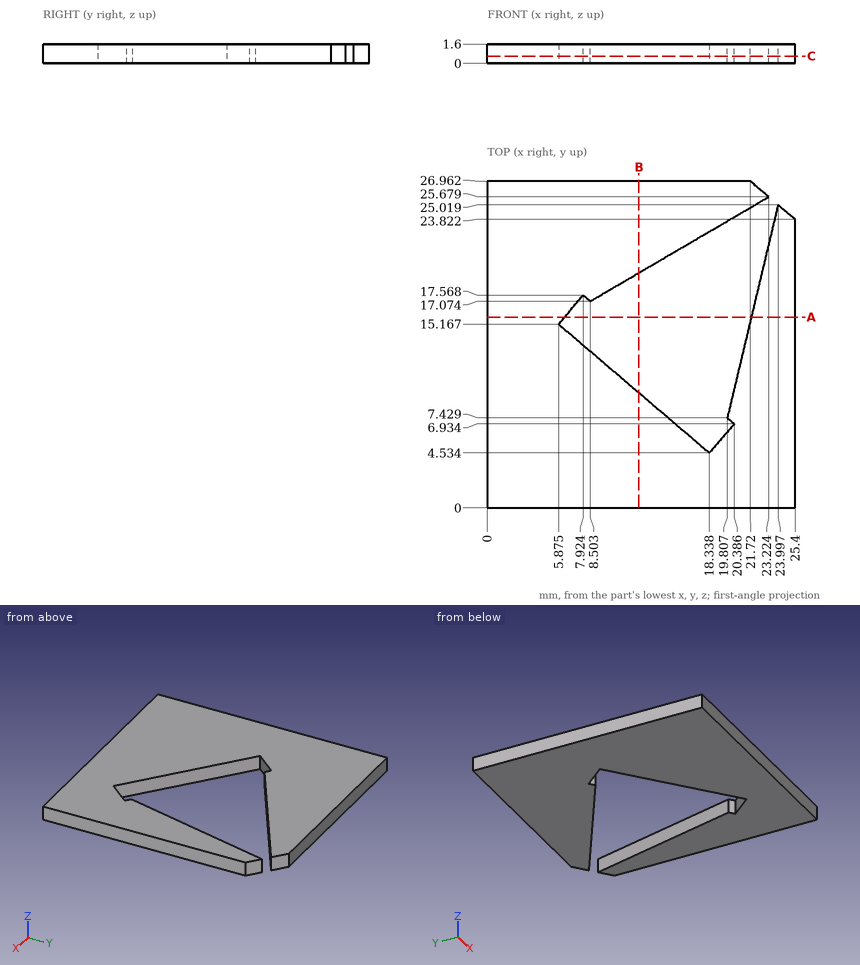
Drawing for the job (mm, zero at the part's lowest x, y, z). Give positions to 0.01 mm unless a question says otherwise; leave off trailing zeros. Loops run counter-clockwise (first coordinate to the right, second up) from the corner with the lowest first, then second, coordinate; pieces in that order, holes last.
(1) Drill centre lines: line 1 along X through (y, z) = (16.5, 0.8) (1 decimal); line 2 along X through (y, z) = (5.25, 1.55); line 3 along Y through (x, z) = (12.75, 0.3) (1 decimal). Where is each one in solid material? Low to high.
Return value:
line 1: x = 0 to 7, 22 to 25.4
line 2: x = 0 to 17.5, 18.95 to 25.4
line 3: y = 0 to 9.3, 19.6 to 27
(2) Band-saw the part on A-A (y = 15.75). Write the cut outline in (x, z).
Return value:
outline: (0, 0) - (6.37, 0) - (6.37, 1.6) - (0, 1.6) - close; (21.79, 0) - (25.4, 0) - (25.4, 1.6) - (21.79, 1.6) - close
(3) Band-saw the part on C-C (z = 0.6). Write the cut outline in (x, y) (1 decimal).
Return value:
outline: (0, 0) - (25.4, 0) - (25.4, 23.8) - (24, 25) - (19.8, 7.4) - (20.4, 6.9) - (18.3, 4.5) - (5.9, 15.2) - (7.9, 17.6) - (8.5, 17.1) - (23.2, 25.7) - (21.7, 27) - (0, 27) - close
(4) Band-saw the part on B-B (x = 12.5). Write the cut outline in (y, z) (1 decimal), and give its area (3 significant figures).
Return value:
outline: (0, 0) - (9.5, 0) - (9.5, 1.6) - (0, 1.6) - close; (19.4, 0) - (27, 0) - (27, 1.6) - (19.4, 1.6) - close
area: 27.3 mm2
